For this review, take the finished solid that the model builds, in its own axes (mm). A direction names the side the tool comes from. Coordinates: 2 decimals unless noted, no trailing zeros. Write each loop counter-clockwise with the first axis right and the second up, starting at its lowest first coordinate (ties: lowest second). Pieces come first, ordered by that corner, then holes.
```python
from build123d import *

# Parameters (mm, degrees)
BOX031_W          = 40
BOX031_H          = 50
BOX031_DEPTH      = 1.4
CYLINDER070_R     = 5
CYLINDER070_DEPTH = 22.75
CYLINDER069_R     = 1.6
CYLINDER069_DEPTH = 22.75
BOX029_W          = 40
BOX029_H          = 50
BOX029_DEPTH      = 10
BOX030_W          = 40
BOX030_H          = 50
BOX030_DEPTH      = 2.3
CYLINDER067_R     = 12.5
CYLINDER067_DEPTH = 7
BOX028_W          = 40
BOX028_H          = 50
BOX028_DEPTH      = 0.7
CYLINDER066_R     = 4
CYLINDER066_DEPTH = 2.75
CYLINDER064_R     = 1.6
CYLINDER064_DEPTH = 22.75
CYLINDER063_R     = 4
CYLINDER063_DEPTH = 2.75
PRISM009_DEPTH    = 3
CYLINDER065_R     = 12.5
CYLINDER065_DEPTH = 7
CHAMFER001_SIZE   = 2.4


with BuildPart() as cube031:
    # Box031 → Box031 (new body)
    with BuildSketch(Plane(origin=(-10, 0, 22.2), x_dir=(1, 0, 0), z_dir=(0, 0, 1))):
        with Locations((20, 25)):
            Rectangle(BOX031_W, BOX031_H)
    extrude(amount=BOX031_DEPTH)


with BuildPart() as cylinder071:
    # Cylinder070 → Cylinder070 (new body)
    with BuildSketch(Plane(origin=(10, 20, 21), x_dir=(1, 0, 0), z_dir=(0, 0, 1))):
        Circle(CYLINDER070_R)
    extrude(amount=CYLINDER070_DEPTH)


with BuildPart() as cylinder070:
    # Cylinder069 → Cylinder069 (new body)
    with BuildSketch(Plane(origin=(10, 20, 12), x_dir=(1, 0, 0), z_dir=(0, 0, 1))):
        Circle(CYLINDER069_R)
    extrude(amount=CYLINDER069_DEPTH)


with BuildPart() as cube029:
    # Box029 → Box029 (new body)
    with BuildSketch(Plane(origin=(-10, 0, 23.5), x_dir=(1, 0, 0), z_dir=(0, 0, 1))):
        with Locations((20, 25)):
            Rectangle(BOX029_W, BOX029_H)
    extrude(amount=BOX029_DEPTH)


with BuildPart() as cube030:
    # Box030 → Box030 (new body)
    with BuildSketch(Plane(origin=(-10, 0, 15.7), x_dir=(1, 0, 0), z_dir=(0, 0, 1))):
        with Locations((20, 25)):
            Rectangle(BOX030_W, BOX030_H)
    extrude(amount=BOX030_DEPTH)


with BuildPart() as cylinder068:
    # Cylinder067 → Cylinder067 (new body)
    with BuildSketch(Plane(origin=(10, 20, 21.5), x_dir=(1, 0, 0), z_dir=(0, 0, 1))):
        Circle(CYLINDER067_R)
    extrude(amount=CYLINDER067_DEPTH)


with BuildPart() as cube028:
    # Box028 → Box028 (new body)
    with BuildSketch(Plane(origin=(-10, 0, 15), x_dir=(1, 0, 0), z_dir=(0, 0, 1))):
        with Locations((20, 25)):
            Rectangle(BOX028_W, BOX028_H)
    extrude(amount=BOX028_DEPTH)


with BuildPart() as cylinder067:
    # Cylinder066 → Cylinder066 (new body)
    with BuildSketch(Plane(origin=(10, 20, 15.2), x_dir=(1, 0, 0), z_dir=(0, 0, 1))):
        Circle(CYLINDER066_R)
    extrude(amount=CYLINDER066_DEPTH)


with BuildPart() as cylinder063:
    # Cylinder064 → Cylinder064 (new body)
    with BuildSketch(Plane(origin=(10, 0, -31), x_dir=(1, 0, 0), z_dir=(0, 0, 1))):
        Circle(CYLINDER064_R)
    extrude(amount=CYLINDER064_DEPTH)


with BuildPart() as cylinder065:
    # Cylinder063 → Cylinder063 (new body)
    with BuildSketch(Plane(origin=(10, 0, -27), x_dir=(1, 0, 0), z_dir=(0, 0, 1))):
        Circle(CYLINDER063_R)
    extrude(amount=CYLINDER063_DEPTH)


with BuildPart() as prism009:
    # Prism009 → Prism009 (new body)
    with BuildSketch(Plane(origin=(10, 0, -20), x_dir=(1, 0, 0), z_dir=(0, 0, -1))):
        Polygon((3.15, 0), (1.575, 2.72798), (-1.575, 2.72798), (-3.15, 0), (-1.575, -2.72798), (1.575, -2.72798), align=None)
    extrude(amount=PRISM009_DEPTH)


with BuildPart() as obj1:
    # Cylinder065 → Cylinder065 (new body)
    with BuildSketch(Plane(origin=(10, 0, -27), x_dir=(1, 0, 0), z_dir=(0, 0, 1))):
        Circle(CYLINDER065_R)
    extrude(amount=CYLINDER065_DEPTH)

    # Cut051: cut Prism009
    add(prism009.part, mode=Mode.SUBTRACT)

    # Cut052: cut Cylinder065
    add(cylinder065.part, mode=Mode.SUBTRACT)

    # Cut053: cut Cylinder063
    add(cylinder063.part, mode=Mode.SUBTRACT)


with BuildPart() as obj1_1:
    # Cut053 placement: moved
    add(obj1.part.moved(Location((0, 20, 42))))

    # Cut055: cut Cylinder067
    add(cylinder067.part, mode=Mode.SUBTRACT)

    # Cut054: cut Cube028
    add(cube028.part, mode=Mode.SUBTRACT)

    # Fusion024: union Cylinder068
    add(cylinder068.part)

    # Cut056: cut Cube030
    add(cube030.part, mode=Mode.SUBTRACT)

    # Cut057: cut Cube029
    add(cube029.part, mode=Mode.SUBTRACT)

    # Cut058: cut Cylinder070
    add(cylinder070.part, mode=Mode.SUBTRACT)

    # Cut059: cut Cylinder071
    add(cylinder071.part, mode=Mode.SUBTRACT)

    # Chamfer001
    chamfer001_edges = [obj1_1.edges().sort_by_distance(p)[0] for p in [
        (5, 20, 23.5),
    ]]
    chamfer(chamfer001_edges, length=CHAMFER001_SIZE)

    # Cut060: cut Cube031
    add(cube031.part, mode=Mode.SUBTRACT)


solid = obj1_1.part
```
Q1. Add section D-D (y = 13). State the section outline as (x, z) points, then the cut area to 3 significant figures.
Ans:
outline: (-0.36, 18) - (20.36, 18) - (20.36, 22.2) - (-0.36, 22.2) - close
area: 87.0 mm2
Q2. Clearance check with flat-ended pins moving along their axes: pin 1 Ø3 at (x, y) = (10, 20) entering from +Z; pin 2 Ø1.5 at (y, z) = (25, 18.5) entering from -X; pin 3 Ø11 at (x, y) = (10, 19.5) entering from +Z; pin 4 Ø4.5 at (x, y) = (11.5, 21.5) entering from +Z. State where each tip first meets the part, or that it passes through.
Ans:
pin 1: passes through
pin 2: stops at x = -1.76
pin 3: stops at z = 22.1
pin 4: stops at z = 21
Q3. Add section A-A (x = 10). State the section outline as (y, z) points, then the cut area to 3 significant figures.
Ans:
outline: (7.5, 18) - (18.4, 18) - (18.4, 19) - (17.27, 19) - (17.27, 21) - (15, 21) - (15, 21.1) - (13.9, 22.2) - (7.5, 22.2) - close; (21.6, 18) - (32.5, 18) - (32.5, 22.2) - (26.1, 22.2) - (25, 21.1) - (25, 21) - (22.73, 21) - (22.73, 19) - (21.6, 19) - close
area: 77.7 mm2
Q4. For probe 1 along X at (y, z) = (20, 18.45); probe 2 along Y at (x, z) = (10, 18.35); probe 3 along X at (y, z) = (20, 21.05), list the stretches that pass through material, from the lowest coordinate up.
Ans:
probe 1: x = -2.5 to 8.4, 11.6 to 22.5
probe 2: y = 7.5 to 18.4, 21.6 to 32.5
probe 3: x = -2.5 to 5, 15 to 22.5
Q5. Add section C-C (y = 27.75). State the section outline as (x, z) points, then the cut area to 3 significant figures.
Ans:
outline: (0.19, 18) - (19.81, 18) - (19.81, 22.2) - (0.19, 22.2) - close
area: 82.4 mm2
Q6. Add section B-B (z = 19.4). State the section outline as (x, y) points (3 decimals), then the cut area to 3 significant figures.
Ans:
outline: circle Ø25 at (10, 20); hole (6.85, 20) - (8.425, 17.272) - (11.575, 17.272) - (13.15, 20) - (11.575, 22.728) - (8.425, 22.728) - close
area: 465 mm2
Q7. Draft analysis for pull direction Y (two halves, no side actions). For faces 3 (the cylindrical face through (0.08, 12.394, 20.071)), 4 (the flat face through (7.649, 18.617, 20.014)), 5 (the flat face through (4, 17, 22.2)), state which applies: +Y half, -Y half, draft (parallel to the pull), parting line (faces both ways), or undercut.
Ans:
face 3: parting line
face 4: undercut
face 5: draft
Q8. Tool access review of faces 1 (the cylindrical face through (9.792, 21.586, 18.493)), 2 (the flat face through (10, 22.728, 20)): name each direction out of +Z, -Z, +X, -X, +Y, -Y from which nothing blocks a thin tool from reaching the whole face with its end or side.
Ans:
face 1: +Z, -Z
face 2: +Z
